Build history of the part. All positions in model axes, mm. Round coordinates to 2 decimals unless told otherwise and drop trailing zeros. Write each loop counter-clockwise with the first axis right and the second up, starting at its lowest first coordinate (ties: lowest second). Pieces come first, ordered by that corner, then holes. Notation, with made-up numbers: M 41.5,85 L 75.5,85 A23 cw 75.5,105 Z; hole C 25.25,-32 d8. An arc over 180 degrees is marked long. Use a Markdown table: item, result.
from build123d import *

# Parameters (mm, degrees)
FRAME_R             = 1.25
FRAME_R_2           = 1.5
FRAME_R_3           = 4
BOSS_EXTRUDE1_DEPTH = 6


with BuildPart() as part:
    # FRAME → Boss-Extrude1 (new body)
    with BuildSketch(Plane.XY):
        Polygon((0, 4.808251585), (0, 365), (5, 370), (365, 370), (370, 365), (370, 5), (365, 0), (345, 0), (343, 2), (339, 6), (333, 6), (329, 2), (41, 2), (37, 6), (31, 6), (27, 2), (25, 0), (5, 0), align=None)
        with Locations((3.295108055, 74.610044833)):
            Circle(FRAME_R, mode=Mode.SUBTRACT)
        with Locations((51.555108055, 150.810044833)):
            Circle(FRAME_R, mode=Mode.SUBTRACT)
        with Locations((3.295108055, 157.160044833)):
            Circle(FRAME_R, mode=Mode.SUBTRACT)
        with Locations((3.295108055, 149.540044833)):
            Circle(FRAME_R, mode=Mode.SUBTRACT)
        with Locations((3.295108055, 124.610044833)):
            Circle(FRAME_R, mode=Mode.SUBTRACT)
        with Locations((51.555108055, 125.880044833)):
            Circle(FRAME_R, mode=Mode.SUBTRACT)
        with Locations((51.555108055, 200.810044833)):
            Circle(FRAME_R, mode=Mode.SUBTRACT)
        with Locations((3.295108055, 207.160044833)):
            Circle(FRAME_R, mode=Mode.SUBTRACT)
        with Locations((50, 6)):
            Circle(FRAME_R_2, mode=Mode.SUBTRACT)
        with Locations((320, 6)):
            Circle(FRAME_R_2, mode=Mode.SUBTRACT)
        with Locations((230, 6)):
            Circle(FRAME_R_2, mode=Mode.SUBTRACT)
        with Locations((140, 6)):
            Circle(FRAME_R_2, mode=Mode.SUBTRACT)
        with Locations((20, 10)):
            Circle(FRAME_R_3, mode=Mode.SUBTRACT)
        with Locations((350, 10)):
            Circle(FRAME_R_3, mode=Mode.SUBTRACT)
        with Locations((10, 40)):
            Circle(FRAME_R_2, mode=Mode.SUBTRACT)
        with Locations((30, 40)):
            Circle(FRAME_R_2, mode=Mode.SUBTRACT)
        with Locations((20, 20)):
            Circle(FRAME_R_2, mode=Mode.SUBTRACT)
        with Locations((350, 20)):
            Circle(FRAME_R_2, mode=Mode.SUBTRACT)
        with Locations((340, 40)):
            Circle(FRAME_R_2, mode=Mode.SUBTRACT)
        with Locations((360, 40)):
            Circle(FRAME_R_2, mode=Mode.SUBTRACT)
        with Locations((360, 360)):
            Circle(FRAME_R_2, mode=Mode.SUBTRACT)
        with Locations((340, 360)):
            Circle(FRAME_R_2, mode=Mode.SUBTRACT)
        with Locations((10, 360)):
            Circle(FRAME_R_2, mode=Mode.SUBTRACT)
        with Locations((30, 360)):
            Circle(FRAME_R_2, mode=Mode.SUBTRACT)
        with Locations((51.555108055, 75.880044833)):
            Circle(FRAME_R, mode=Mode.SUBTRACT)
        with Locations((51.555108055, 68.260044833)):
            Circle(FRAME_R, mode=Mode.SUBTRACT)
        with Locations((5, 269.5)):
            Circle(FRAME_R_2, mode=Mode.SUBTRACT)
        with Locations((48, 269.5)):
            Circle(FRAME_R_2, mode=Mode.SUBTRACT)
        with BuildLine():
            Line((95, 20), (95, 35))
            Line((95, 35), (80, 50))
            Line((80, 50), (60, 50))
            Line((60, 50), (55, 55))
            Line((55, 55), (55, 325))
            Line((55, 325), (60, 330))
            Line((60, 330), (310, 330))
            Line((310, 330), (315, 325))
            Line((315, 325), (315, 55))
            Line((315, 55), (310, 50))
            Line((310, 50), (290, 50))
            Line((290, 50), (275, 35))
            Line((275, 35), (275, 20))
            ThreePointArc((275, 20), (270, 15), (265, 20))
            Line((265, 20), (265, 35))
            Line((265, 35), (260, 40))
            Line((260, 40), (215, 40))
            Line((215, 40), (192.824919816, 17.824919816))
            Line((192.824919816, 17.824919816), (177.175080184, 17.824919816))
            Line((177.175080184, 17.824919816), (155, 40))
            Line((155, 40), (110, 40))
            Line((110, 40), (105, 35))
            Line((105, 35), (105, 20))
            ThreePointArc((105, 20), (100, 15), (95, 20))
        make_face(mode=Mode.SUBTRACT)
    extrude(amount=BOSS_EXTRUDE1_DEPTH)


solid = part.part
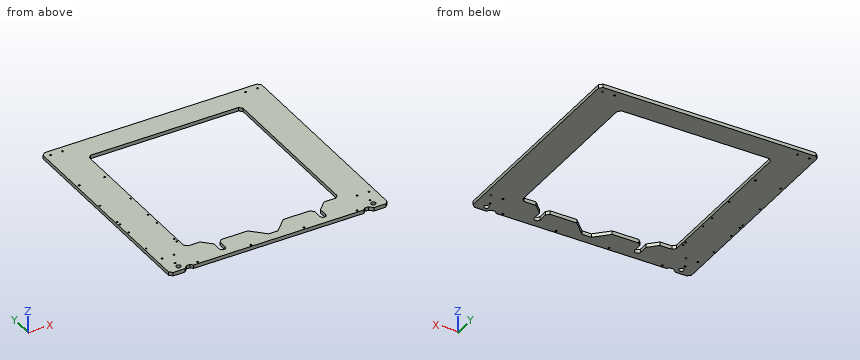
Q1. Drop flat-ended pins along their axis: P1, Ø1, axis at x = 331, z = 3.5, coming from the -Y side; P2, Ø1.8, axis at x = 320, y = 6, coming from the +Z side; P3, Ø1.8, axis at x = 252.5, z = 3, coming from the -Y side. Give the stop position or say it passes through.
Response values:
| item | result |
|---|---|
| P1 | stops at y = 3.5 |
| P2 | passes through |
| P3 | stops at y = 2 |
Q2. Cut at A-A on x = 200. Give the cut face in (y, z).
Response values:
| item | result |
|---|---|
| outline | M 2,0 L 25,0 L 25,6 L 2,6 Z; M 330,0 L 370,0 L 370,6 L 330,6 Z |
Q3. Cut at C-C on z = 1.05. Count the separate pieces of the cut face and the enclosed holes in it, and give its area (3 significant figures).
Response values:
| item | result |
|---|---|
| separate pieces | 1 |
| enclosed holes | 29 |
| area | 59,800 mm2 |
Q4. Drill centre lines: L1, parallel to X at y = 157.5, z = 1.95; L2, parallel to Y at x = 62, z = 2.7; L3, parallel to X at y = 314, z = 3.05. Where is each one in solid material? Low to high.
Response values:
| item | result |
|---|---|
| L1 | x = 0 to 2.09, 4.5 to 55, 315 to 370 |
| L2 | y = 2 to 50, 330 to 370 |
| L3 | x = 0 to 55, 315 to 370 |
Q5. Cut at B-B on y = 181. Give the cut face in (x, z).
Response values:
| item | result |
|---|---|
| outline | M 0,0 L 55,0 L 55,6 L 0,6 Z; M 315,0 L 370,0 L 370,6 L 315,6 Z |
